```python
from build123d import *

# Parameters (mm, degrees)
SKETCH_1_W               = 12
SKETCH_1_H               = 18
EXTRUDE_1_DEPTH          = 12
CUT_EXTRUDE_1_DEPTH      = 12
SKETCH_3_W               = 8
SKETCH_3_H               = 4
CUT_EXTRUDE_2_DEPTH      = 15
EXTRUDE_2_DEPTH          = 4.5
SKETCH_5_W               = 6
SKETCH_5_H               = 9
EXTRUDE_3_DEPTH          = 2.5
FILLET_2_R               = 0.5
CHAMFER_3_SIZE           = 1.5
CHAMFER_4_SIZE           = 1.5
FILLET_3_R               = 1
CUT_EXTRUDE_3_REACH      = 13.5
CUT_EXTRUDE_3_END_RADIUS = 3
CUT_EXTRUDE_4_REACH      = 11.5
CUT_EXTRUDE_4_END_RADIUS = 3
FILLET_6_R               = 1.5
FILLET_7_R               = 1.5


with BuildPart() as part:
    # 草图1 → 拉伸1 (new body)
    with BuildSketch(Plane.XY):
        with Locations((6, 9)):
            Rectangle(SKETCH_1_W, SKETCH_1_H)
    extrude(amount=EXTRUDE_1_DEPTH)

    # 草图2 → 切除-拉伸1 (cut)
    with BuildSketch(Plane.XY.offset(12)):
        with BuildLine():
            Line((3.25, 12.000000088), (3.25, 5.999999721))
            ThreePointArc((3.25, 5.999999721), (6, 3.25), (8.75, 5.999999721))
            Line((8.75, 5.999999721), (8.75, 12.000000088))
            ThreePointArc((8.75, 12.000000088), (6, 14.75), (3.25, 12.000000088))
        make_face()
    extrude(amount=-CUT_EXTRUDE_1_DEPTH, mode=Mode.SUBTRACT)

    # 草图3 → 切除-拉伸2 (cut)
    with BuildSketch(Plane(origin=(0, 18, 0), x_dir=(1, 0, 0), z_dir=(0, 1, 0))):
        with Locations((6, -6)):
            Rectangle(SKETCH_3_W, SKETCH_3_H)
    extrude(amount=-CUT_EXTRUDE_2_DEPTH, mode=Mode.SUBTRACT)

    # 草图4 → 拉伸2 (add)
    with BuildSketch(Plane.XZ):
        with BuildLine():
            Line((9, 10), (6, 10))
            ThreePointArc((6, 10), (3.878679656, 9.121320344), (3, 7))
            Line((3, 7), (3, 4))
            Line((3, 4), (6, 4))
            ThreePointArc((6, 4), (8.121320344, 4.878679656), (9, 7))
            Line((9, 7), (9, 10))
        make_face()
    extrude(amount=EXTRUDE_2_DEPTH)

    # 草图5 → 拉伸3 (add)
    with BuildSketch(Plane.XZ.offset(4.5)):
        with Locations((6, 7)):
            Rectangle(SKETCH_5_W, SKETCH_5_H)
    extrude(amount=-EXTRUDE_3_DEPTH)

    # 圆角2
    fillet_2_edges = [part.edges().sort_by_distance(p)[0] for p in [
        (12, 9, 12),
        (0, 9, 12),
        (12, 9, 0),
        (0, 9, 0),
    ]]
    fillet(fillet_2_edges, radius=FILLET_2_R)

    # 倒角3
    chamfer_3_edges = [part.edges().sort_by_distance(p)[0] for p in [
        (6, -4.5, 11.5),
    ]]
    chamfer(chamfer_3_edges, length=CHAMFER_3_SIZE)

    # 倒角4
    chamfer_4_edges = [part.edges().sort_by_distance(p)[0] for p in [
        (6, -4.5, 2.5),
    ]]
    chamfer(chamfer_4_edges, length=CHAMFER_4_SIZE)

    # 圆角3
    fillet_3_edges = [part.edges().sort_by_distance(p)[0] for p in [
        (6, -4.5, 10),
        (6, -4.5, 4),
    ]]
    fillet(fillet_3_edges, radius=FILLET_3_R)

    # 切除-拉伸3: up to this cylinder (the profile starts outside it)
    cut_extrude_3_end = Plane(origin=(6, -2.105104, 7), z_dir=(0, 1, 0)) * Cylinder(CUT_EXTRUDE_3_END_RADIUS, 34, mode=Mode.PRIVATE)
    # 草图8 → 切除-拉伸3 (cut, up to the surface)
    with BuildSketch(Plane.XY.offset(11.5), mode=Mode.PRIVATE) as cut_extrude_3_sk1:
        Polygon((6, -2), (3, -2), (3, -2.315312706), align=None)
    cut_extrude_3_tool1 = extrude(cut_extrude_3_sk1.sketch, amount=-CUT_EXTRUDE_3_REACH, mode=Mode.PRIVATE) - cut_extrude_3_end
    add(cut_extrude_3_tool1.solids().sort_by_distance((4, -2.105104, 11.5))[0], mode=Mode.SUBTRACT)

    # 切除-拉伸4: up to this cylinder (the profile starts outside it)
    cut_extrude_4_end = Plane(origin=(6, -2.105104, 7), z_dir=(0, 1, 0)) * Cylinder(CUT_EXTRUDE_4_END_RADIUS, 30, mode=Mode.PRIVATE)
    # 草图9 → 切除-拉伸4 (cut, up to the surface)
    with BuildSketch(Plane(origin=(0, 0, 2.5), x_dir=(-1, 0, 0), z_dir=(0, 0, -1)), mode=Mode.PRIVATE) as cut_extrude_4_sk1:
        Polygon((-6, -2), (-9, -2), (-9, -2.315312706), align=None)
    cut_extrude_4_tool1 = extrude(cut_extrude_4_sk1.sketch, amount=-CUT_EXTRUDE_4_REACH, mode=Mode.PRIVATE) - cut_extrude_4_end
    add(cut_extrude_4_tool1.solids().sort_by_distance((8, -2.105104, 2.5))[0], mode=Mode.SUBTRACT)

    # 圆角6
    fillet_6_edges = [part.edges().sort_by_distance(p)[0] for p in [
        (9, -2.657656353, 2.5),
    ]]
    fillet(fillet_6_edges, radius=FILLET_6_R)

    # 圆角7
    fillet_7_edges = [part.edges().sort_by_distance(p)[0] for p in [
        (3, -2.657656353, 11.5),
    ]]
    fillet(fillet_7_edges, radius=FILLET_7_R)


solid = part.part
```
Here's how the part is built. I have some questions about the finished solid (model axes, mm). A direction names the side the tool comes from. Give positions to 0.01 mm unless a question says otherwise; leave off trailing zeros. Order: outer loops, then holes, each group sorted by start corner. A loop starts at its lowest first (then second) coordinate and runs counter-clockwise, first axis right, second up. Notation, with made-up numbers: (-38, 53) -> (-21, 53) arc R21 cw to (-21, 73) -> close; hole circle Ø6 at (39.5, 3.5). An arc over 180 degrees is marked (long way). Use CSV: the item, a comma, the result in double quotes. Start each with the question number.
Item 1: Thinking about a two-plate mould opening in Y: for faces 1 (the flat face through (6, -4.5, 7)), 2 (the cylindrical face through (6.06, 14.75, 2.03)), 3 (the flat face through (2, 9, 0)), 4 (the flat face through (8.75, 9, 2)), which applies, pulls with the +Y half, pulls with the -Y half, needs draft (parallel to the pull), parting line crosses it, or undercut?
Item 2: Suppose I cut it at A-A (z = 1). List the corners of the cut face in (x, y) for me.
Item 3: If I drill on probe 1 along Z at (x, y) = (3, 16); probe 2 along X at (y, z) = (15.5, 6.5); probe 3 along X at (y, z) = (6, 2.25), over which ranges is the centre line in solid material (lowest first)? Write a range as [from, to].
Item 4: Suppose I cut it at D-D (z = 5). List the corners of the cut face in (x, y) for me.
Item 5: On a 3-axis mill with a long thin cutter (end or side, diameter ignored), from which of +Z, -Z, +X, -X, +Y, -Y can I reach the whole of each face in a straight line? I mean faces 5 (the cylindrical face through (5.94, 3.25, 2.03)), 6 (the cylindrical face through (8.1, -1.14, 4.86)), 7 (the flat face through (9, -3, 8)), 8 (the cylindrical face through (3.3, -3, 10.9)), 9 (the flat face through (3, 14, 8)). Say none if no direction works.
Item 6: Suppose I cut it at C-C (x = 2.75). List the corners of the cut face in (y, z) for me.
Item 7: Suppose I cut it at B-B (y = 4). List the corners of the cut face in (x, z) for me, and give its area (3 significant figures).
Item 8: I'm going to push flat-ended pins straight in: P1, Ø3.5, axis at y = -2, z = 7.5, coming from the -X side; P2, Ø2, axis at x = 5, y = 8.5, coming from the +Z side; P3, Ø1.2, axis at x = 5, z = 6, coming from the +Y side; P4, Ø2, axis at x = 1.5, z = 10, coming from the -Y side. Where does each tip first touch, or does it pass through?
Answer block:
1,face 1,"pulls with the -Y half"
1,face 2,"undercut"
1,face 3,"needs draft"
1,face 4,"undercut"
2,outline,"(0, 0) -> (12, 0) -> (12, 18) -> (0, 18) -> close; hole (3.25, 6) arc R2.75 ccw to (8.75, 6) -> (8.75, 12) arc R2.75 ccw to (3.25, 12) -> close"
3,probe 1,"z = [0, 4], [8, 12]"
3,probe 2,"x = [0, 2], [10, 12]"
3,probe 3,"x = [0, 3.25], [8.75, 12]"
4,outline,"(0, 0) -> (3, 0) -> (3, -4.5) -> (9, -4.5) -> (9, -2.32) -> (8.24, -2.24) -> (8.24, 0) -> (12, 0) -> (12, 18) -> (10, 18) -> (10, 3) -> (2, 3) -> (2, 18) -> (0, 18) -> close"
5,face 5,"+Z, -Z"
5,face 6,"-Z, +X"
5,face 7,"+Z, -Z, +X, -Y"
5,face 8,"+Z, -X, -Y"
5,face 9,"+Y"
6,outline,"(0, 0) -> (18, 0) -> (18, 4) -> (3, 4) -> (3, 8) -> (18, 8) -> (18, 12) -> (0, 12) -> close"
7,outline,"(0, 0.5) arc R0.5 ccw to (0.5, 0) -> (4.11, 0) -> (4.11, 4) -> (2, 4) -> (2, 8) -> (4.11, 8) -> (4.11, 12) -> (0.5, 12) arc R0.5 ccw to (0, 11.5) -> close; (7.89, 0) -> (11.5, 0) arc R0.5 ccw to (12, 0.5) -> (12, 11.5) arc R0.5 ccw to (11.5, 12) -> (7.89, 12) -> (7.89, 8) -> (10, 8) -> (10, 4) -> (7.89, 4) -> close"
7,area,"81.6 mm^2"
8,P1,"stops at x = 3"
8,P2,"passes through"
8,P3,"stops at y = 3"
8,P4,"stops at y = 0"
